Work out the finished part from the listing and answer in its coordinate system (mm). Face numbers are marked on the shaded views. A direction names the side the tool comes from. Give positions to 0.01 mm unless a question says otherwise; leave off trailing zeros. Write each loop counter-clockwise with the first axis right and the second up, starting at its lowest first coordinate (ties: lowest second). Pieces come first, ordered by that corner, then holes. Notation, with made-up numbers: (33.25, 37) - (83.25, 37) arc R17 ccw to (83.25, 63) - close; hole circle Ø5 at (25, 4). An arc over 180 degrees is marked (long way). Write each question's results on one line, items separated by ' | '. Start each with the question number.
from build123d import *

# Parameters (mm, degrees)
BOSS_EXTRUDE1_DEPTH      = 2.6
BOSS_EXTRUDE1_DEPTH_BACK = 6
SKETCH3_W                = 50
SKETCH3_H                = 66.691620804
BOSS_EXTRUDE2_DEPTH      = 4
SKETCH8_R                = 2.1
CUT_EXTRUDE4_DEPTH       = 63.560770456
CHAMFER1_SIZE            = 2.5
SKETCH9_W                = 37
SKETCH9_H                = 5
BOSS_EXTRUDE3_DEPTH      = 34.5
SKETCH10_R               = 1.6
CUT_EXTRUDE5_DEPTH       = 74.011642907
BOSS_EXTRUDE4_DEPTH      = 3
CHAMFER2_SIZE            = 3


with BuildPart() as part:
    # Sketch3 → Boss-Extrude1 (new, two sides: drawn at the far end of the back side and taken through both)
    with BuildSketch(Plane.XY.offset(-BOSS_EXTRUDE1_DEPTH_BACK)):
        with Locations((0, 5.654189598)):
            Rectangle(SKETCH3_W, SKETCH3_H)
    extrude(amount=BOSS_EXTRUDE1_DEPTH + BOSS_EXTRUDE1_DEPTH_BACK)

    # Sketch7 → Boss-Extrude2 (add)
    with BuildSketch(Plane(origin=(0, 0, -6), x_dir=(-1, 0, 0), z_dir=(0, 0, -1))):
        with BuildLine():
            Line((-25, 39), (-3.663721376, 55.451541401))
            ThreePointArc((-3.663721376, 55.451541401), (0, 56.7), (3.663721376, 55.451541401))
            Line((3.663721376, 55.451541401), (25, 39))
            Line((25, 39), (-25, 39))
        make_face()
    extrude(amount=-BOSS_EXTRUDE2_DEPTH)

    # Sketch8 → Cut-Extrude4 (cut, through all)
    with BuildSketch(Plane.XY.offset(2.6)):
        with Locations((-19, 5.7)):
            Circle(SKETCH8_R)
        with Locations((19, 5.7)):
            Circle(SKETCH8_R)
        with Locations((0, 50.7)):
            Circle(SKETCH8_R)
    extrude(amount=-CUT_EXTRUDE4_DEPTH, mode=Mode.SUBTRACT)

    # Chamfer1
    chamfer1_edges = [part.edges().sort_by_distance(p)[0] for p in [
        (-21.1, 5.7, 2.6),
        (16.9, 5.7, 2.6),
        (-2.1, 50.7, -2),
    ]]
    chamfer(chamfer1_edges, length=CHAMFER1_SIZE)

    # Sketch9 → Boss-Extrude3 (add)
    with BuildSketch(Plane.XY.offset(2.6)):
        with Locations((0, -3.5)):
            Rectangle(SKETCH9_W, SKETCH9_H)
    extrude(amount=BOSS_EXTRUDE3_DEPTH)

    # Sketch10 → Cut-Extrude5 (cut, through all)
    with BuildSketch(Plane(origin=(0, -1, 0), x_dir=(1, 0, 0), z_dir=(0, 1, 0))):
        with Locations(Location((9.75, -13.35, 0), (0, 0, 270))):
            Circle(SKETCH10_R)
        with Locations(Location((9.75, -32.85, 0), (0, 0, 270))):
            Circle(SKETCH10_R)
        with Locations(Location((-9.75, -32.85, 0), (0, 0, 270))):
            Circle(SKETCH10_R)
        with Locations(Location((-9.75, -13.35, 0), (0, 0, 270))):
            Circle(SKETCH10_R)
        with BuildLine():
            Line((-5, -23.1), (-5, -37.1))
            Line((-5, -37.1), (5, -37.1))
            Line((5, -37.1), (5, -23.1))
            ThreePointArc((5, -23.1), (0, -18.1), (-5, -23.1))
        make_face()
    extrude(amount=-CUT_EXTRUDE5_DEPTH, mode=Mode.SUBTRACT)

    # Sketch11 → Boss-Extrude4 (add)
    with BuildSketch(Plane.ZY.offset(18.5)):
        Polygon((2.6, -1), (2.6, 1), (37.1, -1), align=None)
        Polygon((2.6, -6), (2.6, -27.691620804), (37.1, -6), align=None)
    boss_extrude4 = extrude(amount=-BOSS_EXTRUDE4_DEPTH)

    # Mirror1: Boss-Extrude4 across plane
    add(boss_extrude4.mirror(Plane(origin=(0, 0, 0), x_dir=(0, 0, 1), z_dir=(1, 0, 0))))

    # Chamfer2
    # the kernel refuses this chamfer: 3 mm, written as the material it takes off along each edge
    with BuildSketch(Plane(origin=(9.75, -6, 32.85), x_dir=(0, 0, 1), z_dir=(-1, 0, 0))) as chamfer2_piece_1:
        Polygon((1.6 + CHAMFER2_SIZE, 0), (1.6, CHAMFER2_SIZE), (1.6, 0), align=None)
    revolve(axis=Axis((9.75, -6, 32.85), (0, 1, 0)), mode=Mode.SUBTRACT)
    with BuildSketch(Plane(origin=(-9.75, -6, 32.85), x_dir=(0, 0, 1), z_dir=(-1, 0, 0))) as chamfer2_piece_2:
        Polygon((1.6 + CHAMFER2_SIZE, 0), (1.6, CHAMFER2_SIZE), (1.6, 0), align=None)
    revolve(axis=Axis((-9.75, -6, 32.85), (0, 1, 0)), mode=Mode.SUBTRACT)
    with BuildSketch(Plane(origin=(-9.75, -6, 13.35), x_dir=(0, 0, 1), z_dir=(-1, 0, 0))) as chamfer2_piece_3:
        Polygon((1.6 + CHAMFER2_SIZE, 0), (1.6, CHAMFER2_SIZE), (1.6, 0), align=None)
    revolve(axis=Axis((-9.75, -6, 13.35), (0, 1, 0)), mode=Mode.SUBTRACT)
    with BuildSketch(Plane(origin=(9.75, -6, 13.35), x_dir=(0, 0, 1), z_dir=(-1, 0, 0))) as chamfer2_piece_4:
        Polygon((1.6 + CHAMFER2_SIZE, 0), (1.6, CHAMFER2_SIZE), (1.6, 0), align=None)
    revolve(axis=Axis((9.75, -6, 13.35), (0, 1, 0)), mode=Mode.SUBTRACT)


solid = part.part
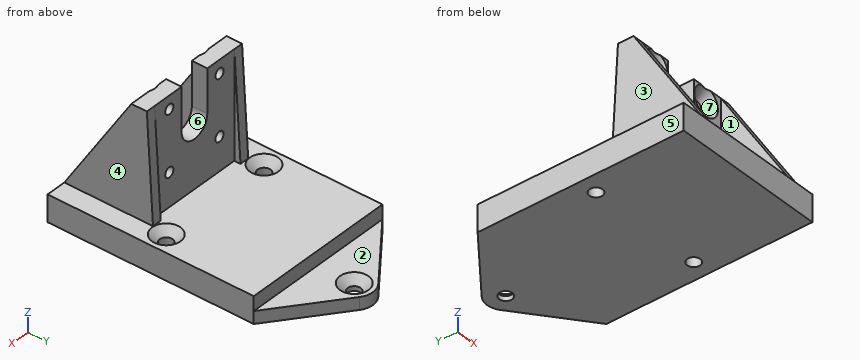
Q1. Consider L1, parallel to X at y = -2.1, z = 32.85; L2, parallel to X at y = -1.8, z = 13.35; L3, parallel to X at y = -9.5, z = 29. Determine where each line is inside the solid, lowest interval first.
Q2. A cutting plane is placed at D-D, the plane y = 50.7. Write down the section's boundary in (x, z), and give its area (3 significant figures).
Q3. The mould has two halves that part along Z. Classify the marked faces 5, 6 and 7: pulls with the +Z half, pulls with the -Z half, needs draft (parallel to the pull), parting line crosses it, or undercut.
Q4. Given pin 1 (11 mm diameter, centred on x = -2.5, y = -15, fed in from +Z); pin 2 (1 mm diameter, centred on y = -13.5, z = 17.5, fed in from +X); pin 3 (2 mm diameter, centred on x = 7.5, z = 16.5, fed in from +Y); pin 4 (1.9 mm diameter, centred on x = 9.75, z = 13.35, fed in from -Y), each flat-ended and moving along its own axis, determine where each tip first touches the part or whether it passes through.
Q5. A cutting plane is placed at B-B, the plane x = 0. Write down the section's boundary in (y, z), and give its area (3 significant figures).
Q6. A cutting plane is placed at C-C, the plane z = 19. Write down the section's boundary in (x, y).
Q7. A tool of negligible diameter and unlimited length cuts with its end or side. For the marked faces 1, 2, 3 and 4, from which of +Z, -Z, +X, -X, +Y, -Y can it reach the whole face along a straight path? Write none if from no direction.
Q8. A cutting plane is placed at A-A, the plane y = 5.7. Write down the section's boundary in (x, z).
Result:
1) L1: x = -18.5 to -11.35, -8.15 to -5, 5 to 8.15, 11.35 to 18.5 | L2: x = -18.5 to -11.35, -8.15 to 8.15, 11.35 to 18.5 | L3: x = -18.5 to -15.5, 15.5 to 18.5
2) outline: (-9.83, -6) - (-2.1, -6) - (-2.1, -4.5) - (-4.6, -2) - (-9.83, -2) - close; (2.1, -6) - (9.83, -6) - (9.83, -2) - (4.6, -2) - (2.1, -4.5) - close | area: 55.6 mm2
3) face 5: needs draft | face 6: pulls with the +Z half | face 7: undercut
4) pin 1: stops at z = 2.6 | pin 2: stops at x = 18.5 | pin 3: stops at y = -1 | pin 4: passes through
5) outline: (-27.69, -6) - (48.6, -6) - (48.6, -4.5) - (46.1, -2) - (39, -2) - (39, 2.6) - (-1, 2.6) - (-1, 18.1) - (-6, 18.1) - (-6, 2.6) - (-27.69, 2.6) - close; (52.8, -6) - (56.7, -6) - (56.7, -2) - (55.3, -2) - (52.8, -4.5) - close | area: 699 mm2
6) outline: (-18.5, -17.38) - (-15.5, -17.38) - (-15.5, -6) - (-2.86, -6) - (-2.86, -1) - (-15.5, -1) - (-15.5, 0.05) - (-18.5, 0.05) - close; (2.86, -6) - (15.5, -6) - (15.5, -17.38) - (18.5, -17.38) - (18.5, 0.05) - (15.5, 0.05) - (15.5, -1) - (2.86, -1) - close
7) face 1: +Z, -Y | face 2: +Z, +X, -X, +Y | face 3: +Z, -X, +Y, -Y | face 4: +Z, +X, +Y, -Y
8) outline: (-25, -6) - (-21.1, -6) - (-21.1, 0.1) - (-23.6, 2.6) - (-25, 2.6) - close; (-16.9, -6) - (16.9, -6) - (16.9, 0.1) - (14.4, 2.6) - (-14.4, 2.6) - (-16.9, 0.1) - close; (21.1, -6) - (25, -6) - (25, 2.6) - (23.6, 2.6) - (21.1, 0.1) - close
